```python
from build123d import *

# Parameters (mm, degrees)
F0_W     = 184.15
F0_H     = 101.6
F1_DEPTH = 114.3
F2_W     = 82.55
F2_H     = 88.9
F3_DEPTH = 107.95
F5_DEPTH = 101.601
F6_R     = 7.62
F7_R     = 19.05
F8_DEPTH = 25.4


with BuildPart() as f1:
    # F0 (on Top) → F1 (new body)
    with BuildSketch(Plane.XY):
        with Locations((-5.291667, -7.821875)):
            Rectangle(F0_W, F0_H)
    extrude(amount=F1_DEPTH)

    # F2 (on face) → F3 (cut)
    with BuildSketch(Plane.XY.offset(114.3)):
        with Locations((-49.741667, -7.821875)):
            Rectangle(F2_W, F2_H)
        with Locations((39.158333, -7.821875)):
            Rectangle(F2_W, F2_H)
    extrude(amount=-F3_DEPTH, mode=Mode.SUBTRACT)

    # F4 (on face) → F5 (cut, through all)
    with BuildSketch(Plane.XZ.offset(58.621875)):
        Polygon((-97.366667, 114.3), (-97.366667, 38.1), (86.783333, 114.3), align=None)
    extrude(amount=-F5_DEPTH, mode=Mode.SUBTRACT)

    # F6
    f6_edges = [f1.edges().sort_by_distance(p)[0] for p in [
        (80.433333, 36.628125, 59.011207),
        (-8.466667, 36.628125, 40.618103),
        (-97.366667, 42.978125, 19.05),
        (-97.366667, -58.621875, 19.05),
        (86.783333, -58.621875, 57.15),
        (80.433333, -52.271875, 59.011207),
        (-8.466667, -52.271875, 40.618103),
        (86.783333, 42.978125, 57.15),
        (-2.116667, -52.271875, 41.931897),
        (-91.016667, -52.271875, 23.538793),
        (-2.116667, 36.628125, 41.931897),
        (-91.016667, 36.628125, 23.538793),
    ]]
    fillet(f6_edges, radius=F6_R)

    # F7 (on face) → F8 (cut)
    with BuildSketch(Plane(origin=(-97.366667, 0, 0), x_dir=(0, -1, 0), z_dir=(-1, 0, 0))):
        with Locations((7.821875, 38.1)):
            Circle(F7_R)
    extrude(amount=-F8_DEPTH, mode=Mode.SUBTRACT)


solid = f1.part
```
Design review of the part built by this model. Coordinates are the model's own, in mm. A direction names the side the tool comes from. Give positions to 0.01 mm unless a question says otherwise; leave off trailing zeros. Loops run counter-clockwise (first coordinate to the right, second up) from the corner with the lowest first, then second, coordinate; pieces in that order, holes last. Notation, with made-up numbers: (-9, -3) -> (21, -3) arc R16 cw to (21, 5) -> close; hole circle Ø11 at (33, 74.5). An arc over 180 degrees is marked (long way). Write each question's results on one line, items separated by ' | '.
Q1. The part is to be moulded in two halves that separate along X. For faces 1 (the face through (-95.19, 40.69, 20.92)), 2 (the face through (-10.758, 34.455, 40.138)), 3 (the face through (12, -58.622, 42)), say which applies: +X half, -X half, draft (parallel to the pull), parting line (faces both ways), or undercut.
Reply:
face 1: -X half | face 2: undercut | face 3: draft
Q2. Take a section at C-C, the plane x = 61. Write out the cut boundary in (y, z), plus the area to 3 significant figures.
Reply:
outline: (-58.62, 0) -> (42.98, 0) -> (42.98, 103.63) -> (36.63, 103.63) -> (36.63, 6.35) -> (-52.27, 6.35) -> (-52.27, 103.63) -> (-58.62, 103.63) -> close | area: 1,880 mm²
Q3. Take a section at B-B, the plane z = 23.5. Write out the cut boundary in (x, y).
Reply:
outline: (-97.37, -51) arc R7.62 ccw to (-89.75, -58.62) -> (79.16, -58.62) arc R7.62 ccw to (86.78, -51) -> (86.78, 35.36) arc R7.62 ccw to (79.16, 42.98) -> (-89.75, 42.98) arc R7.62 ccw to (-97.37, 35.36) -> (-97.37, 4.42) -> (-91.02, 4.42) -> (-91.02, 29.01) arc R7.62 cw to (-83.4, 36.63) -> (-16.09, 36.63) arc R7.62 cw to (-8.47, 29.01) -> (-8.47, -44.65) arc R7.62 cw to (-16.09, -52.27) -> (-83.4, -52.27) arc R7.62 cw to (-91.02, -44.65) -> (-91.02, -20.06) -> (-97.37, -20.06) -> close; hole (-2.12, -44.65) arc R7.62 ccw to (5.5, -52.27) -> (72.81, -52.27) arc R7.62 ccw to (80.43, -44.65) -> (80.43, 29.01) arc R7.62 ccw to (72.81, 36.63) -> (5.5, 36.63) arc R7.62 ccw to (-2.12, 29.01) -> close
Q4. Wall thickness on L1, parallel to X at y = -36, z = 22.5; L2, parallel to Y at x = -21, z = 68; L3, parallel to X at y = 0, z = 64: over which ranges is each line inside the solid? List them lowest first.
Reply:
L1: x = -97.37 to -91.02, -8.47 to -2.12, 80.43 to 86.78 | L2: y = -58.62 to -52.27, 36.63 to 42.98 | L3: x = -8.47 to -2.12, 80.43 to 86.78
Q5. For pin 1 Ø23 at (y, z) = (-7.82, 38.1) entering from -X; pin 2 Ø4 at (x, y) = (-8.5, -37.5) entering from +Z, all flat-tipped, find the tip position at first contact; note any pin that passes through.
Reply:
pin 1: stops at x = -8.47 | pin 2: stops at z = 75.7
Q6. Machinability: for faces 4 (the face through (-50, -7, 6.35)), 5 (the face through (-95.194, -56.33, 20.915)), which of the approach directions +Z, -Z, +X, -X, +Y, -Y give a long, thin tool a straight path to every point of the face, cutting with its end or side? Answer none if there is none.
Reply:
face 4: +Z | face 5: +Z, -Z, -X, -Y
Q7. Take a section at D-D, the plane z = 94. Write out the cut boundary in (x, y) (3 decimals), plus the area to 3 significant figures.
Reply:
outline: (37.725, -58.622) -> (79.163, -58.622) arc R7.62 ccw to (86.783, -51.002) -> (86.783, 35.358) arc R7.62 ccw to (79.163, 42.978) -> (37.725, 42.978) -> (37.725, 36.628) -> (72.813, 36.628) arc R7.62 cw to (80.433, 29.008) -> (80.433, -44.652) arc R7.62 cw to (72.813, -52.272) -> (37.725, -52.272) -> close | area: 1,190 mm²
Q8. Take a section at A-A, the plane y = -40. Write out the cut boundary in (x, z), plus the area to 3 significant figures.
Reply:
outline: (-97.37, 0) -> (86.78, 0) -> (86.78, 114.3) -> (80.43, 111.67) -> (80.43, 6.35) -> (-2.12, 6.35) -> (-2.12, 77.51) -> (-8.47, 74.89) -> (-8.47, 6.35) -> (-91.02, 6.35) -> (-91.02, 40.73) -> (-97.37, 38.1) -> close | area: 2,500 mm²
